Design review of the part built by this model. Coordinates are the model's own, in mm. A direction names the side the tool comes from. Coordinates: 2 decimals unless noted, no trailing zeros. Order: outer loops, then holes, each group sorted by start corner. A loop starts at its lowest first (then second) coordinate and runs counter-clockwise, first axis right, second up.
from build123d import *

# Parameters (mm, degrees)
SKETCH1_R           = 4.05
BOSS_EXTRUDE1_DEPTH = 10
SKETCH2_R           = 5.55
SKETCH2_R_2         = 4.05
BOSS_EXTRUDE2_DEPTH = 2.5
FILLET1_R           = 1


with BuildPart() as part:
    # Sketch1 → Boss-Extrude1 (new body)
    with BuildSketch(Plane.XY):
        Polygon((8.65, -4.994079828), (8.65, 4.994079828), (0, 9.988159657), (-8.65, 4.994079828), (-8.65, -4.994079828), (0, -9.988159657), align=None)
        Circle(SKETCH1_R, mode=Mode.SUBTRACT)
    extrude(amount=BOSS_EXTRUDE1_DEPTH)

    # Sketch2 → Boss-Extrude2 (add)
    with BuildSketch(Plane.XY.offset(10)):
        Circle(SKETCH2_R)
        Circle(SKETCH2_R_2, mode=Mode.SUBTRACT)
    extrude(amount=BOSS_EXTRUDE2_DEPTH)

    # Fillet1
    fillet1_edges = [part.edges().sort_by_distance(p)[0] for p in [
        (-4.05, 0, 0),
        (-5.55, 0, 10),
        (-4.325, -7.491119743, 0),
        (-8.65, 0, 0),
        (-4.325, 7.491119743, 0),
        (4.325, 7.491119743, 0),
        (8.65, 0, 0),
        (4.325, -7.491119743, 0),
    ]]
    fillet(fillet1_edges, radius=FILLET1_R)


solid = part.part
1. Insertion check: pin 1 (1.5 mm diameter, centred on x = 3.5, z = 4.5, fed in from +Y). The pin has a flat end and moves straight along its axis. Give the tip position at first contact, or say it passes through.
2. Mouldability with a two-part tool opening along Y and no side actions: class faces 3 (the cylindrical face through (2.98, 4.68, 11.74)), 4 (the cylindrical face through (-8.349, -0.07, 0.285)), 5 (the cylindrical face through (-0.878, -3.954, 6.67)), 6 (the cylindrical face through (-4.114, -7.266, 0.285)) as pulls with the +Y half, pulls with the -Y half, needs draft (parallel to the pull), parting line crosses it, or undercut.
3. To check wall thickness, follow line 1 (Z direction, x = -6.75, y = -3); line 2 (Z direction, x = -3.75, y = -3.25); line 3 (X direction, y = 1.75, z = 1.75). State the ranges of each line that lie inside material, in increasing order.
4. For faces 1 (the flat face through (0, -7, 10)), 2 (the cylindrical face through (8.349, 0.07, 0.285)), list the 3-axis set-ups (+Z, -Z, +X, -X, +Y, -Y) from which the entire face can be reached by the end or side of a thin tool; tool diameter is ignored.
5. Add section A-A (y = 0). Give the boundary of the cut face in (x, z).
6. Add section B-B (z = 5.5). Give the boundary of the cut face in (x, y), and give its area (3 significant figures).
Solution:
1. pin 1: stops at y = 8.4
2. face 3: parting line crosses it
2. face 4: needs draft
2. face 5: undercut
2. face 6: pulls with the -Y half
3. line 1: z = 0 to 10
3. line 2: z = 0 to 12.5
3. line 3: x = -8.65 to -3.65, 3.65 to 8.65
4. face 1: +Z
4. face 2: -Z, +X, +Y, -Y
5. outline: (-8.65, 1) arc R1 ccw to (-7.65, 0) - (-5.05, 0) arc R1 ccw to (-4.05, 1) - (-4.05, 12.5) - (-5.55, 12.5) - (-5.55, 11) arc R1 cw to (-6.55, 10) - (-8.65, 10) - close; (4.05, 1) arc R1 ccw to (5.05, 0) - (7.65, 0) arc R1 ccw to (8.65, 1) - (8.65, 10) - (6.55, 10) arc R1 cw to (5.55, 11) - (5.55, 12.5) - (4.05, 12.5) - close
6. outline: (-8.65, -4.99) - (0, -9.99) - (8.65, -4.99) - (8.65, 4.99) - (0, 9.99) - (-8.65, 4.99) - close; hole circle Ø8.1 at (0, 0)
6. area: 208 mm2
